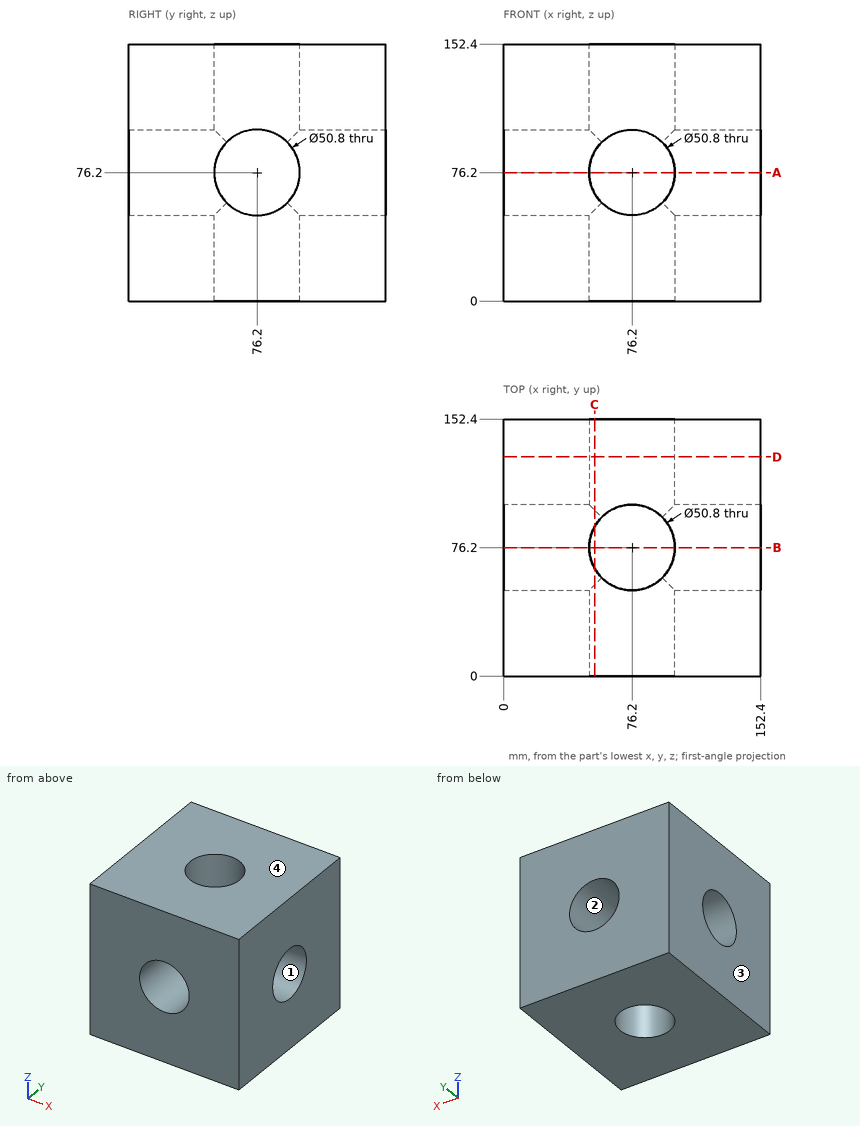
Input: dimensioned drawing with shaded views. Units: mm. Origin: part minimum x, y, z. Round coordinates to 2 decimals unless told otherwise and drop trailing zeros. Order: outer loops, then holes, each group sorted by start corner. A loop starts at its lowest first (then second) coordinate and runs counter-clockwise, first axis right, second up. Notation, with made-up numbers: M -13,37 L 41,37 A15 cw 41,49 Z; hole C 32,-23.5 d9. An arc over 180 degrees is marked long. Use one line per item in the form item = value. Start each with the question number.
Q1. Cut plane C-C (x = 54). Return loops of the section in (y, z), and give its area (3 significant figures).
Q2. Material intervals for line 1 (Y direction, x = 120.5, z = 76.2); line 2 (X direction, y = 92, z = 127), sorted ascending. Write a range as [from, to].
Q3. Mould query, pull axis Z, two halves, no side actions, for the marked faces 1, 2, 3 and 4. Classes: +Z half, -Z half, draft (parallel to the pull), parting line (faces both ways), or undercut.
Q4. Cut plane A-A (z = 76.2). Return loops of the section in (x, y).
Q5. Pin query (flat end, axial travel): pin 1 Ø10 at (x, z) = (106.5, 45) entering from -Y. Return the tip coordinate at first contact, or that it passes through.
Q6. Cut plane D-D (y = 130). Return loops of the section in (x, z).
Geometry results:
q1.outline = M 0,0 L 63.86,0 L 63.86,54 A25.4 cw 54,63.86 L 0,63.86 Z; M 0,88.54 L 54,88.54 A25.4 cw 63.86,98.4 L 63.86,152.4 L 0,152.4 Z; M 88.54,0 L 152.4,0 L 152.4,63.86 L 98.4,63.86 A25.4 cw 88.54,54 Z; M 88.54,98.4 A25.4 cw 98.4,88.54 L 152.4,88.54 L 152.4,152.4 L 88.54,152.4 Z
q1.area = 16,100 mm^2
q2.line_1 = [0, 50.8], [101.6, 152.4]
q2.line_2 = [0, 56.31], [96.09, 152.4]
q3.face_1 = undercut
q3.face_2 = undercut
q3.face_3 = draft
q3.face_4 = +Z half
q4.outline = M 0,0 L 50.8,0 L 50.8,50.8 L 0,50.8 Z; M 0,101.6 L 50.8,101.6 L 50.8,152.4 L 0,152.4 Z; M 101.6,0 L 152.4,0 L 152.4,50.8 L 101.6,50.8 Z; M 101.6,101.6 L 152.4,101.6 L 152.4,152.4 L 101.6,152.4 Z
q5.pin_1 = 0
q6.outline = M 0,0 L 152.4,0 L 152.4,152.4 L 0,152.4 Z; hole C 76.2,76.2 d50.8
